The listing builds one solid part. Answer for the finished solid, in the listing's coordinates (mm). A direction names the side the tool comes from. Round coordinates to 2 decimals unless told otherwise and drop trailing zeros. Write each loop counter-clockwise with the first axis right and the second up, starting at its lowest first coordinate (ties: lowest second). Pieces come first, ordered by that corner, then holes.
(1) The mould has two halves that part along X. Classify faces 3 (the face through (-14.6, -11.93, 13.58)), 4 (the face through (0, -15, 14)), 5 (the face through (-11.4, 11.93, 13.58)), 6 (the face through (-2.93, -13.18, 9.16)): +X half, -X half, draft (parallel to the pull), parting line (faces both ways), or undercut.
(2) Each of these flat-tipped pins is pushed along its axis until it touches: pin 1 Ø1.5 at (x, z) = (3, 7) entering from +Y; pin 2 Ø8 at (y, z) = (0.5, 5.5) entering from -X; pin 3 Ø2 at (y, z) = (-6, 2.5) entering from -X. Where does it stop, or does it pass through?
(3) For faces 1 (the face through (11.923, 3.755, 3.106)), 2 (the face through (11.4, 12.07, 13.58)), determine the directions among +Z, -Z, +X, -X, +Y, -Y from which every point of the face is accessible in a straight line to the end or side of a thin tool.
(4) A cutting plane is placed at D-D, the plane y = 11.5. Give the vertices of the cut face in (x, z).
(5) Find the intervals of material crossed by probe 1 along Y at (x, z) = (-13, 13.5); probe 2 along Y at (x, z) = (0, 11.5); probe 3 along Y at (x, z) = (1, 4.25), in increasing order.
(6) A cutting plane is placed at A-A, the plane y = 0. Give the vertices of the cut face in (x, z).
(7) A cutting plane is placed at B-B, the plane x = -3. Give the vertices of the cut face in (y, z).
(8) A cutting plane is placed at C-C, the plane z = 13.25. Give the vertices of the cut face in (x, y), and give its area (3 significant figures).
from build123d import *

# Parameters (mm, degrees)
SKETCH_1_R      = 12.5
SKETCH_1_R_2    = 9
EXTRUDE_1_DEPTH = 6.3
SKETCH_2_R      = 13.5
SKETCH_2_R_2    = 9
EXTRUDE_2_DEPTH = 5.8
SKETCH_3_W      = 36
SKETCH_3_H      = 30
SKETCH_3_R      = 9
SKETCH_3_R_2    = 1.6
EXTRUDE_3_DEPTH = 3
FILLET_1_R      = 3


with BuildPart() as part:
    # 草图1 → 凸台-拉伸1 (new body)
    with BuildSketch(Plane.XY):
        Circle(SKETCH_1_R)
        Circle(SKETCH_1_R_2, mode=Mode.SUBTRACT)
    extrude(amount=EXTRUDE_1_DEPTH)

    # 草图2 → 凸台-拉伸2 (add)
    with BuildSketch(Plane.XY.offset(6.3)):
        Circle(SKETCH_2_R)
        Circle(SKETCH_2_R_2, mode=Mode.SUBTRACT)
    extrude(amount=EXTRUDE_2_DEPTH)

    # 草图3 → 凸台-拉伸3 (add)
    with BuildSketch(Plane.XY.offset(12.1)):
        Rectangle(SKETCH_3_W, SKETCH_3_H)
        Circle(SKETCH_3_R, mode=Mode.SUBTRACT)
        with Locations((13, 12)):
            Circle(SKETCH_3_R_2, mode=Mode.SUBTRACT)
        with Locations(Location((13, -12, 0), (0, 0, 180))):
            Circle(SKETCH_3_R_2, mode=Mode.SUBTRACT)
        with Locations((-13, -12)):
            Circle(SKETCH_3_R_2, mode=Mode.SUBTRACT)
        with Locations(Location((-13, 12, 0), (0, 0, 180))):
            Circle(SKETCH_3_R_2, mode=Mode.SUBTRACT)
    extrude(amount=EXTRUDE_3_DEPTH)

    # 圆角1
    fillet_1_edges = [part.edges().sort_by_distance(p)[0] for p in [
        (18, 15, 13.6),
        (-18, 15, 13.6),
        (-18, -15, 13.6),
        (18, -15, 13.6),
    ]]
    fillet(fillet_1_edges, radius=FILLET_1_R)


solid = part.part
Solutions:
1. face 3: undercut
1. face 4: draft
1. face 5: undercut
1. face 6: parting line
2. pin 1: stops at y = 13.31
2. pin 2: stops at x = -13.5
2. pin 3: stops at x = -11.46
3. face 1: -Z
3. face 2: +Z, -Z
4. outline: (-18, 12.1) - (-14.52, 12.1) - (-14.52, 15.1) - (-18, 15.1) - close; (-11.48, 12.1) - (-7.07, 12.1) - (-7.07, 6.3) - (-4.9, 6.3) - (-4.9, 0) - (4.9, 0) - (4.9, 6.3) - (7.07, 6.3) - (7.07, 12.1) - (11.48, 12.1) - (11.48, 15.1) - (-11.48, 15.1) - close; (14.52, 12.1) - (18, 12.1) - (18, 15.1) - (14.52, 15.1) - close
5. probe 1: y = -15 to -13.6, -10.4 to 10.4, 13.6 to 15
5. probe 2: y = -13.5 to -9, 9 to 13.5
5. probe 3: y = -12.46 to -8.94, 8.94 to 12.46
6. outline: (-18, 12.1) - (-13.5, 12.1) - (-13.5, 6.3) - (-12.5, 6.3) - (-12.5, 0) - (-9, 0) - (-9, 15.1) - (-18, 15.1) - close; (9, 0) - (12.5, 0) - (12.5, 6.3) - (13.5, 6.3) - (13.5, 12.1) - (18, 12.1) - (18, 15.1) - (9, 15.1) - close
7. outline: (-15, 12.1) - (-13.16, 12.1) - (-13.16, 6.3) - (-12.13, 6.3) - (-12.13, 0) - (-8.49, 0) - (-8.49, 15.1) - (-15, 15.1) - close; (8.49, 0) - (12.13, 0) - (12.13, 6.3) - (13.16, 6.3) - (13.16, 12.1) - (15, 12.1) - (15, 15.1) - (8.49, 15.1) - close
8. outline: (-18, -12) arc R3 ccw to (-15, -15) - (15, -15) arc R3 ccw to (18, -12) - (18, 12) arc R3 ccw to (15, 15) - (-15, 15) arc R3 ccw to (-18, 12) - close; hole circle Ø3.2 at (-13, -12); hole circle Ø3.2 at (-13, 12); hole circle Ø18 at (0, 0); hole circle Ø3.2 at (13, -12); hole circle Ø3.2 at (13, 12)
8. area: 786 mm2
